```python
from build123d import *

# Parameters (mm, degrees)
F0_W     = 130
F0_H     = 105
F1_DEPTH = 5
F4_DEPTH = 25
F5_W     = 11.439742
F5_H     = 95.512622
F6_DEPTH = 25


with BuildPart() as f1:
    # F0 (on Top) → F1 (new body)
    with BuildSketch(Plane.XY):
        Rectangle(F0_W, F0_H)
    extrude(amount=F1_DEPTH)

    # F3 (on face) → F4 (join)
    with BuildSketch(Plane(origin=(0, 0, 0), x_dir=(1, 0, 0), z_dir=(0, 0, -1))):
        Polygon((57.5, 33.844031), (57.5, -33.844031), (57.5, -52.5), (65, -52.5), (65, 52.5), (57.5, 52.5), align=None)
        Polygon((-57.5, -52.5), (-57.5, -33.844031), (-57.5, 33.844031), (-57.5, 52.5), (-65, 52.5), (-65, -52.5), align=None)
    extrude(amount=F4_DEPTH)

    # F5 (on face) → F6 (cut)
    with BuildSketch(Plane.XY.offset(5)):
        Rectangle(F5_W, F5_H)
        with Locations((25, 0)):
            Rectangle(F5_W, F5_H)
        with Locations((50, 0)):
            Rectangle(F5_W, F5_H)
        with Locations((-25, 0)):
            Rectangle(F5_W, F5_H)
        with Locations((-50, 0)):
            Rectangle(F5_W, F5_H)
    extrude(amount=-F6_DEPTH, mode=Mode.SUBTRACT)


solid = f1.part
```
The listing builds one solid part. Answer for the finished solid, in the listing's coordinates (mm). A direction names the side the tool comes from. Coordinates: 2 decimals unless noted, no trailing zeros. Loops run counter-clockwise (first coordinate to the right, second up) from the corner with the lowest first, then second, coordinate; pieces in that order, holes last. Notation, with made-up numbers: (-17, 57.5) - (40, 57.5) arc R23 cw to (40, 71.5) - close; hole circle Ø1 at (0.5, 23). An arc over 180 degrees is marked (long way). Write item = value, one per line.
1) Section D-D (z = 2.5) is taken. Determine the outline of the cut face in (x, y).
Responses:
outline = (-65, -52.5) - (65, -52.5) - (65, 52.5) - (-65, 52.5) - close; hole (-55.72, -47.76) - (-44.28, -47.76) - (-44.28, 47.76) - (-55.72, 47.76) - close; hole (-30.72, -47.76) - (-19.28, -47.76) - (-19.28, 47.76) - (-30.72, 47.76) - close; hole (-5.72, -47.76) - (5.72, -47.76) - (5.72, 47.76) - (-5.72, 47.76) - close; hole (19.28, -47.76) - (30.72, -47.76) - (30.72, 47.76) - (19.28, 47.76) - close; hole (44.28, -47.76) - (55.72, -47.76) - (55.72, 47.76) - (44.28, 47.76) - close
2) Which of the six approach directions +Z, -Z, +X, -X, +Y, -Y give full straight-line access (tool end or side, diameter ignored) to faces 1 (the face through (-14, 1, 0)), 2 (the face through (-19.28, -1, 3)), 3 (the face through (61, -1, -25))?
Responses:
face_1 = -Z, +Y, -Y
face_2 = +Z, -Z
face_3 = -Z, +X, -X, +Y, -Y
3) Find the intervals of material crossed by line 1 along X through (y, z) = (40.5, 1.75); line 2 along X through (y, z) = (7, -12.5); line 3 along Z through (x, y) = (17, 26.5), in increasing order.
Responses:
line_1 = -65 to -55.72, -44.28 to -30.72, -19.28 to -5.72, 5.72 to 19.28, 30.72 to 44.28, 55.72 to 65
line_2 = -65 to -57.5, 57.5 to 65
line_3 = 0 to 5
4) Section A-A (z = -4) is taken. Determine the outline of the cut face in (x, y), plus the area to 4 significant figures.
Responses:
outline = (-65, -52.5) - (-57.5, -52.5) - (-57.5, 52.5) - (-65, 52.5) - close; (57.5, -52.5) - (65, -52.5) - (65, 52.5) - (57.5, 52.5) - close
area = 1,575 mm^2
5) This flat-tipped pin is pushed along its axis until it touches: P1, Ø1.5, axis at x = 32, y = -11, coming from the -Z side. Where does it stop, or does it pass through?
Responses:
P1 = 0
6) Section B-B (y = 8) is taken. Determine the outline of the cut face in (x, z).
Responses:
outline = (-65, -25) - (-57.5, -25) - (-57.5, 0) - (-55.72, 0) - (-55.72, 5) - (-65, 5) - close; (-44.28, 0) - (-30.72, 0) - (-30.72, 5) - (-44.28, 5) - close; (-19.28, 0) - (-5.72, 0) - (-5.72, 5) - (-19.28, 5) - close; (5.72, 0) - (19.28, 0) - (19.28, 5) - (5.72, 5) - close; (30.72, 0) - (44.28, 0) - (44.28, 5) - (30.72, 5) - close; (55.72, 0) - (57.5, 0) - (57.5, -25) - (65, -25) - (65, 5) - (55.72, 5) - close
7) Section C-C (x = -2) is taken. Determine the outline of the cut face in (y, z).
Responses:
outline = (-52.5, 0) - (-47.76, 0) - (-47.76, 5) - (-52.5, 5) - close; (47.76, 0) - (52.5, 0) - (52.5, 5) - (47.76, 5) - close
8) Determine the mould class of faces 4 (the face through (-65, -1, -10)), 5 (the face through (-30.72, -1, 3)), 6 (the face through (19.28, -1, 3)) for opening direction Y: pulls with the +Y half, pulls with the -Y half, needs draft (parallel to the pull), parting line crosses it, or undercut.
Responses:
face_4 = needs draft
face_5 = undercut
face_6 = undercut
